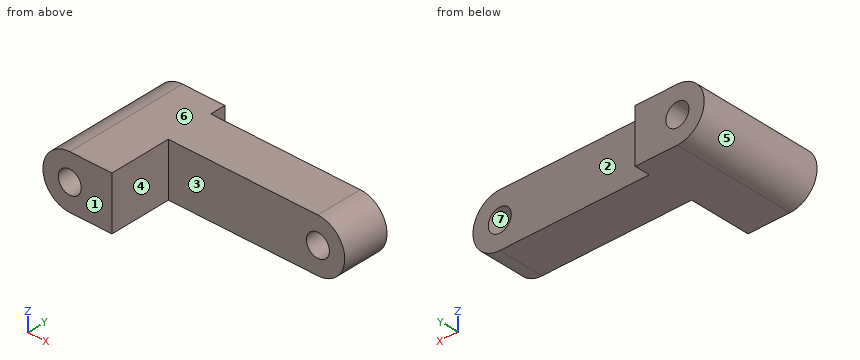
```python
from build123d import *

# Parameters (mm, degrees)
F0_R     = 1.5
F1_DEPTH = 8
F2_W     = 40.742426
F2_H     = 15.659974
F2_W_2   = 45.289567
F2_H_2   = 22.391903
F3_DEPTH = 25.4


with BuildPart() as f1:
    # F0 (on Front) → F1 (new body, symmetric)
    with BuildSketch(Plane.XZ):
        with BuildLine():
            ThreePointArc((14, 0), (12.5, 1.5), (11, 0))
            ThreePointArc((11, 0), (12.5, -1.5), (14, 0))
        make_face()
        with Locations((-12.5, 0)):
            Circle(F0_R)
        with BuildLine():
            Line((12.5, 3.5), (-12.5, 3.5))
            ThreePointArc((-12.5, 3.5), (-16, 0), (-12.5, -3.5))
            Line((-12.5, -3.5), (12.5, -3.5))
            ThreePointArc((12.5, -3.5), (16, 0), (12.5, 3.5))
        make_face()
        with Locations((-12.5, 0)):
            Circle(F0_R, mode=Mode.SUBTRACT)
        with BuildLine():
            ThreePointArc((14, 0), (12.5, -1.5), (11, 0))
            ThreePointArc((11, 0), (12.5, 1.5), (14, 0))
        make_face(mode=Mode.SUBTRACT)
    extrude(amount=F1_DEPTH, both=True)

    # F2 (on face) → F3 (cut)
    with BuildSketch(Plane.XY.offset(3.5)):
        with Locations((13.371213, 13.829987)):
            Rectangle(F2_W, F2_H)
        with Locations((15.644783, -11.195951)):
            Rectangle(F2_W_2, F2_H_2)
    extrude(amount=-F3_DEPTH, mode=Mode.SUBTRACT)


solid = f1.part
```
Build history of the part. All positions in model axes, mm. Face numbers are marked on the shaded views. A direction names the side the tool comes from. Coordinates: 2 decimals unless noted, no trailing zeros. Order: outer loops, then holes, each group sorted by start corner. A loop starts at its lowest first (then second) coordinate and runs counter-clockwise, first axis right, second up. Notation, with made-up numbers: M -23,71.25 L -7,71.25 A25 ccw -7,91.25 Z; hole C 44,73 d7. An arc over 180 degrees is marked long. One line per question, with ' | ' between items. Start each with the question number.
1. Cut at B-B (y = -3.25). Write the cut outline in (x, z), plus the area to 3 significant figures.
2. Wall check: line 1 along Z through (x, y) = (12.5, 1.4); line 2 along X through (y, z) = (1, -1); line 3 along X through (y, z) = (-1.25, 0.75). Give the ranges that are in metal, low to high. Write a range as [from, to].
3. Cut at D-D (z = 3). Write the cut outline in (x, y), plus the area to 3 significant figures.
4. Cut at C-C (y = 1.75). Write the cut outline in (x, z).
5. Flat gauge pins, fed straight in: P1, Ø1.6, axis at y = 7, z = 1, coming from the +X side; P2, Ø1.5, axis at x = -1.5, z = 1, coming from the +Y side; P3, Ø1.5, axis at y = -0.5, z = -1, coming from the -X side. Where does each tip first touch, or does it go through?
6. Tool access for the marked faces 1, 2 and 3: list every direction of +Z, -Z, +X, -X, +Y, -Y with a clear straight run to the whole face (end or side of a thin tool).
7. Mould opens along X. For the marked faces 4, 5, 6 and 7 say: +X half, -X half, draft (parallel to the pull), parting line (faces both ways), or undercut.
8. Cut at A-A (z = 0). Write the cut outline in (x, y).
The answers:
1) outline: M -12.5,-3.5 L -7,-3.5 L -7,3.5 L -12.5,3.5 A3.5 ccw Z; hole C -12.5,0 d3 | area: 50.7 mm2
2) line 1: z = [-3.5, -1.5], [1.5, 3.5] | line 2: x = [-15.85, -13.62], [-11.38, 11.38], [13.62, 15.85] | line 3: x = [-15.92, -13.8], [-11.2, -7]
3) outline: M -14.3,-8 L -7,-8 L -7,0 L 14.3,0 L 14.3,6 L -7,6 L -7,8 L -14.3,8 Z | area: 245 mm2
4) outline: M -12.5,-3.5 L 12.5,-3.5 A3.5 ccw 12.5,3.5 L -12.5,3.5 A3.5 ccw Z; hole C -12.5,0 d3; hole C 12.5,0 d3
5) P1: stops at x = -7 | P2: stops at y = 6 | P3: stops at x = -15.99
6) face 1: +Z, -Z, +X, -X, -Y | face 2: +Z, -Z, +X, +Y | face 3: +Z, -Z, +X, -Y
7) face 4: +X half | face 5: -X half | face 6: draft | face 7: undercut
8) outline: M -16,-8 L -14,-8 L -14,8 L -16,8 Z; M -11,-8 L -7,-8 L -7,0 L 11,0 L 11,6 L -7,6 L -7,8 L -11,8 Z; M 14,0 L 16,0 L 16,6 L 14,6 Z
